Verification items for the finished model (mm, model axes). A direction names the side the tool comes from. Coordinates: 2 decimals unless noted, no trailing zeros. Write each loop counter-clockwise with the first axis right and the second up, starting at its lowest first coordinate (ties: lowest second). Pieces come first, ordered by that corner, then holes. Notation, with made-up numbers: M -34,54 L -15,54 A8 ccw -15,61 Z; hole C 45,59 d10. An arc over 180 degrees is marked long. Answer in a Markdown table with one row per item.
from build123d import *

# Parameters (mm, degrees)
BOSS_EXTRUDE1_DEPTH = 508
SKETCH3_W           = 304.8
SKETCH3_H           = 203.2
CUT_EXTRUDE3_DEPTH  = 6.35
SHELL2_START        = 6.35
SHELL2_DEPTH        = 495.3
CUT_EXTRUDE5_REACH  = 881.882


# Read off the part's stored shape, not the designer's step: Shell2
with BuildPart() as part:
    # Sketch1 → Boss-Extrude1 (new body)
    with BuildSketch(Plane.XY):
        Polygon((0, 101.6), (0, 609.6), (282.846955047, 609.6), (508, 288.048127639), (508, 101.6), align=None)
    extrude(amount=BOSS_EXTRUDE1_DEPTH)

    # Sketch3 → Cut-Extrude3 (cut)
    with BuildSketch(Plane(origin=(-2211.042315979, 4171.242991451, 0), x_dir=(0, 0, -1), z_dir=(-0.8191520442889911, -0.573576436351047, 0))):
        with Locations((-254, 4544.813258204)):
            Rectangle(SKETCH3_W, SKETCH3_H)
    extrude(amount=CUT_EXTRUDE3_DEPTH, mode=Mode.SUBTRACT)

    # Shell2 outline → Shell2 (cut)
    with BuildSketch(Plane.XY.offset(SHELL2_START)):
        Polygon((501.65, 107.95), (501.65, 286.045980329), (279.541354276, 603.25), (6.35, 603.25), (6.35, 107.95), align=None)
    extrude(amount=SHELL2_DEPTH, mode=Mode.SUBTRACT)

    # Sketch10 → Cut-Extrude5 (cut, up to next)
    with BuildSketch(Plane(origin=(0, 609.6, 0), x_dir=(1, 0, 0), z_dir=(0, 1, 0)), mode=Mode.PRIVATE) as cut_extrude5_sk1:
        with BuildLine():
            Line((143.381985017, -385.451435914), (144.181985017, -385.451435914))
            ThreePointArc((144.181985017, -385.451435914), (145.596198579, -386.037222352), (146.181985017, -387.451435914))
            Line((146.181985017, -387.451435914), (146.181985017, -408.951435914))
            ThreePointArc((146.181985017, -408.951435914), (145.596198579, -410.365649476), (144.181985017, -410.951435914))
            Line((144.181985017, -410.951435914), (143.381985017, -410.951435914))
            ThreePointArc((143.381985017, -410.951435914), (141.967771454, -410.365649476), (141.381985017, -408.951435914))
            Line((141.381985017, -408.951435914), (141.381985017, -387.451435914))
            ThreePointArc((141.381985017, -387.451435914), (141.967771454, -386.037222352), (143.381985017, -385.451435914))
        make_face()
    cut_extrude5_tool1 = extrude(cut_extrude5_sk1.sketch, amount=-CUT_EXTRUDE5_REACH, mode=Mode.PRIVATE) & part.part
    # Sketch10 → Cut-Extrude5 (cut, up to next)
    with BuildSketch(Plane(origin=(0, 609.6, 0), x_dir=(1, 0, 0), z_dir=(0, 1, 0)), mode=Mode.PRIVATE) as cut_extrude5_sk2:
        with BuildLine():
            Line((144.181985017, -312.438871317), (143.381985017, -312.438871317))
            ThreePointArc((143.381985017, -312.438871317), (141.967771454, -311.853084879), (141.381985017, -310.438871317))
            Line((141.381985017, -310.438871317), (141.381985017, -288.938871317))
            ThreePointArc((141.381985017, -288.938871317), (141.967771454, -287.524657755), (143.381985017, -286.938871317))
            Line((143.381985017, -286.938871317), (144.181985017, -286.938871317))
            ThreePointArc((144.181985017, -286.938871317), (145.596198579, -287.524657755), (146.181985017, -288.938871317))
            Line((146.181985017, -288.938871317), (146.181985017, -310.438871317))
            ThreePointArc((146.181985017, -310.438871317), (145.596198579, -311.853084879), (144.181985017, -312.438871317))
        make_face()
    cut_extrude5_tool2 = extrude(cut_extrude5_sk2.sketch, amount=-CUT_EXTRUDE5_REACH, mode=Mode.PRIVATE) & part.part
    # Sketch10 → Cut-Extrude5 (cut, up to next)
    with BuildSketch(Plane(origin=(0, 609.6, 0), x_dir=(1, 0, 0), z_dir=(0, 1, 0)), mode=Mode.PRIVATE) as cut_extrude5_sk3:
        with BuildLine():
            Line((144.181985017, -213.92630672), (143.381985017, -213.92630672))
            ThreePointArc((143.381985017, -213.92630672), (141.967771454, -213.340520282), (141.381985017, -211.92630672))
            Line((141.381985017, -211.92630672), (141.381985017, -190.42630672))
            ThreePointArc((141.381985017, -190.42630672), (141.967771454, -189.012093158), (143.381985017, -188.42630672))
            Line((143.381985017, -188.42630672), (144.181985017, -188.42630672))
            ThreePointArc((144.181985017, -188.42630672), (145.596198579, -189.012093158), (146.181985017, -190.42630672))
            Line((146.181985017, -190.42630672), (146.181985017, -211.92630672))
            ThreePointArc((146.181985017, -211.92630672), (145.596198579, -213.340520282), (144.181985017, -213.92630672))
        make_face()
    cut_extrude5_tool3 = extrude(cut_extrude5_sk3.sketch, amount=-CUT_EXTRUDE5_REACH, mode=Mode.PRIVATE) & part.part
    # Sketch10 → Cut-Extrude5 (cut, up to next)
    with BuildSketch(Plane(origin=(0, 609.6, 0), x_dir=(1, 0, 0), z_dir=(0, 1, 0)), mode=Mode.PRIVATE) as cut_extrude5_sk4:
        with BuildLine():
            Line((144.181985017, -115.413742123), (143.381985017, -115.413742123))
            ThreePointArc((143.381985017, -115.413742123), (141.967771454, -114.827955685), (141.381985017, -113.413742123))
            Line((141.381985017, -113.413742123), (141.381985017, -91.913742123))
            ThreePointArc((141.381985017, -91.913742123), (141.967771454, -90.499528561), (143.381985017, -89.913742123))
            Line((143.381985017, -89.913742123), (144.181985017, -89.913742123))
            ThreePointArc((144.181985017, -89.913742123), (145.596198579, -90.499528561), (146.181985017, -91.913742123))
            Line((146.181985017, -91.913742123), (146.181985017, -113.413742123))
            ThreePointArc((146.181985017, -113.413742123), (145.596198579, -114.827955685), (144.181985017, -115.413742123))
        make_face()
    cut_extrude5_tool4 = extrude(cut_extrude5_sk4.sketch, amount=-CUT_EXTRUDE5_REACH, mode=Mode.PRIVATE) & part.part
    add(cut_extrude5_tool1.solids().sort_by_distance((143.781985, 609.6, 398.201436))[0], mode=Mode.SUBTRACT)
    add(cut_extrude5_tool2.solids().sort_by_distance((143.781985, 609.6, 299.688871))[0], mode=Mode.SUBTRACT)
    add(cut_extrude5_tool3.solids().sort_by_distance((143.781985, 609.6, 201.176307))[0], mode=Mode.SUBTRACT)
    add(cut_extrude5_tool4.solids().sort_by_distance((143.781985, 609.6, 102.663742))[0], mode=Mode.SUBTRACT)


solid = part.part
1) Release check for a two-part mould opening along Y. For faces 3 (the face through (468.9, 343.89, 250.44)), 4 (the face through (508, 196, 250)), 5 (the face through (501.65, 196, 251)) record: +Y half, -Y half, draft (parallel to the pull), parting line (faces both ways), or undercut.
Response values:
| item | result |
|---|---|
| face 3 | +Y half |
| face 4 | draft |
| face 5 | undercut |
2) Tool access check on faces 1 (the face through (139, 609.6, 250)), 2 (the face through (318.114, 548.162, 250.533)). Record the directions out of +Z, -Z, +X, -X, +Y, -Y that give a thin tool (end or side, any length) a straight path to the whole face; none if there is none.
Response values:
| item | result |
|---|---|
| face 1 | +Z, -Z, +X, -X, +Y |
| face 2 | none |
3) Depth check by flat-ended pin: pin 1 (3 mm diameter, centred on y = 608, z = 204.5, fed in from +X); pin 2 (3 mm diameter, centred on y = 547.5, z = 273.5, fed in from +X); pin 3 (10 mm diameter, centred on y = 373.5, z = 332.5, fed in from +X). Enter the tip coordinate at first touch or a pass-through.
Response values:
| item | result |
|---|---|
| pin 1 | stops at x = 285.02 |
| pin 2 | stops at x = 327.38 |
| pin 3 | stops at x = 6.35 |
4) Sectioned sample at B-B (y = 270). Record the cut outline in (x, z), then the cut area to 3 significant figures.
Response values:
| item | result |
|---|---|
| outline | M 0,0 L 508,0 L 508,508 L 0,508 Z; hole M 6.35,6.35 L 501.65,6.35 L 501.65,501.65 L 6.35,501.65 Z |
| area | 12,700 mm² |
5) Sectioned sample at C-C (x = 211). Record the cut outline in (y, z).
Response values:
| item | result |
|---|---|
| outline | M 101.6,0 L 609.6,0 L 609.6,508 L 101.6,508 Z; hole M 107.95,6.35 L 603.25,6.35 L 603.25,501.65 L 107.95,501.65 Z |
6) Sectioned sample at D-D (z = 82.5). Record the cut outline in (x, y), then the cut area to 3 significant figures.
Response values:
| item | result |
|---|---|
| outline | M 0,101.6 L 508,101.6 L 508,288.05 L 282.85,609.6 L 0,609.6 Z; hole M 6.35,107.95 L 501.65,107.95 L 501.65,286.05 L 279.54,603.25 L 6.35,603.25 Z |
| area | 11,800 mm² |
7) Thickness scan on L1, parallel to Z at x = 212.5, y = 498; L2, parallel to Y at x = 94, z = 361.5. Record the ranges inside material, lowest first. Write a range as [from, to].
Response values:
| item | result |
|---|---|
| L1 | z = [0, 6.35], [501.65, 508] |
| L2 | y = [101.6, 107.95], [603.25, 609.6] |
8) Sectioned sample at A-A (z = 321.5). Record the cut outline in (x, y), then the cut area to 3 significant figures.
Response values:
| item | result |
|---|---|
| outline | M 0,101.6 L 508,101.6 L 508,288.05 L 454.03,365.12 L 448.83,361.48 L 501.65,286.05 L 501.65,107.95 L 6.35,107.95 L 6.35,603.25 L 279.54,603.25 L 332.28,527.93 L 337.48,531.58 L 282.85,609.6 L 0,609.6 Z |
| area | 10,500 mm² |
